Check sheet for the modelled part. Datum: model origin and axes. Units: mm. Face numbers are marked on the shaded views. Round coordinates to 2 decimals unless told otherwise and drop trailing zeros. Write each loop counter-clockwise with the first axis right and the second up, starting at its lowest first coordinate (ties: lowest second). Pieces come first, ordered by that corner, then holes. Notation, with made-up numbers: M 14,72 L 57,72 A17 cw 57,85 Z; hole C 64,67 d10. An arc over 180 degrees is marked long. Answer in a Markdown table with one row per item.
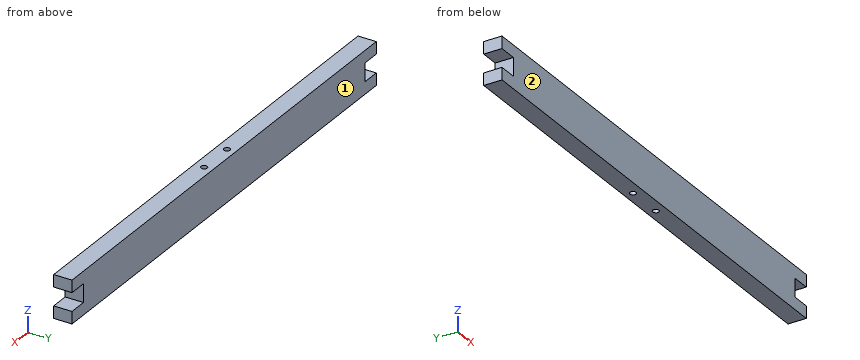
```python
from build123d import *

# Parameters (mm, degrees)
EXTRUDE_1_DEPTH     = 15
SKETCH_4_R          = 2.5
CUT_EXTRUDE_1_DEPTH = 35


with BuildPart() as part:
    # 草图3 → 凸台-拉伸1 (new body)
    with BuildSketch(Plane(origin=(0, 0, 0), x_dir=(1, 0, 0), z_dir=(0, 1, 0))):
        Polygon((0, 0), (400, 0), (400, 10), (385, 10), (385, 25), (400, 25), (400, 35), (0, 35), (0, 25), (15, 25), (15, 10), (0, 10), align=None)
    extrude(amount=EXTRUDE_1_DEPTH)

    # 草图4 → 切除-拉伸1 (cut)
    with BuildSketch(Plane.XY):
        with Locations((185, 8)):
            Circle(SKETCH_4_R)
        with Locations((215, 8)):
            Circle(SKETCH_4_R)
    extrude(amount=-CUT_EXTRUDE_1_DEPTH, mode=Mode.SUBTRACT)


solid = part.part
```
1. Go/stop test with flat-tipped pins: pin 1 (4.5 mm diameter, centred on x = 185, y = 8, fed in from -Z); pin 2 (1.5 mm diameter, centred on y = 8, z = -21, fed in from -X). Record where each tip stops, or that it passes through.
Found:
| item | result |
|---|---|
| pin 1 | passes through |
| pin 2 | stops at x = 15 |
2. Scan lines: L1, parallel to X at y = 8.5, z = -29.5; L2, parallel to X at y = 8.5, z = -17.5; L3, parallel to Y at x = 185, z = -21. Record each from-to range of solid material in increasing order.
Found:
| item | result |
|---|---|
| L1 | x = 0 to 182.55, 187.45 to 212.55, 217.45 to 400 |
| L2 | x = 15 to 182.55, 187.45 to 212.55, 217.45 to 385 |
| L3 | y = 0 to 5.5, 10.5 to 15 |
3. Draft check along Y on the marked faces 1 and 2. Enter one of: +Y half, -Y half, draft (parallel to the pull), parting line (faces both ways), or undercut.
Found:
| item | result |
|---|---|
| face 1 | +Y half |
| face 2 | -Y half |
4. Section check A-A, the plane y = 8. Record the cut outline in (x, z), and give its area (3 significant figures).
Found:
| item | result |
|---|---|
| outline | M 0,-35 L 182.5,-35 L 182.5,0 L 0,0 L 0,-10 L 15,-10 L 15,-25 L 0,-25 Z; M 187.5,-35 L 212.5,-35 L 212.5,0 L 187.5,0 Z; M 217.5,-35 L 400,-35 L 400,-25 L 385,-25 L 385,-10 L 400,-10 L 400,0 L 217.5,0 Z |
| area | 13,200 mm2 |
